Work out the finished part from the listing and answer in its coordinate system (mm). A direction names the side the tool comes from. Give positions to 0.01 mm unless a question says otherwise; leave off trailing zeros. Write each loop counter-clockwise with the first axis right and the second up, starting at its lowest first coordinate (ties: lowest second). Pieces come first, ordered by that corner, then holes. Notation, with made-up numbers: (45.5, 53) - (73.5, 53) arc R4 ccw to (73.5, 59) - close; hole circle Ø5 at (89.25, -13.75). An arc over 180 degrees is marked (long way). Write each question's results on one line, items separated by ' | '. Start each with the question number.
from build123d import *

# Parameters (mm, degrees)
ESQUISSE2_R             = 8.85
ESQUISSE2_R_2           = 8
ENL_V_MAT_EXTRU_1_DEPTH = 8
ESQUISSE3_R             = 1.5
ENL_V_MAT_EXTRU_2_DEPTH = 7
ESQUISSE4_R             = 1
ENL_V_MAT_EXTRU_3_DEPTH = 10
ESQUISSE6_R             = 1
ENL_V_MAT_EXTRU_4_DEPTH = 10
ESQUISSE7_R             = 1
ENL_V_MAT_EXTRU_5_DEPTH = 10


with BuildPart() as part:
    # Esquisse1 → Révolution1 (revolve)
    with BuildSketch(Plane.XY, mode=Mode.PRIVATE) as r_volution1_sk:
        Polygon((2.5, 0), (13.9, 0), (13.9, 1.5), (12.4, 1.5), (12.4, 8), (13.9, 8), (13.9, 9.5), (8.85, 9.5), (8.85, 17.5), (2.5, 17.5), align=None)
    revolve(r_volution1_sk.sketch.rotate(Axis((0, 0, 0), (0, 1, 0)), 90), axis=Axis((0, 0, 0), (0, 1, 0)))

    # Esquisse2 → Enlèv. mat.-Extru.1 (cut)
    with BuildSketch(Plane(origin=(0, 17.5, 0), x_dir=(1, 0, 0), z_dir=(0, 1, 0))):
        Circle(ESQUISSE2_R)
        with Locations(Location((0, 0, 0), (0, 0, 270))):
            Circle(ESQUISSE2_R_2, mode=Mode.SUBTRACT)
    extrude(amount=-ENL_V_MAT_EXTRU_1_DEPTH, mode=Mode.SUBTRACT)

    # Esquisse3 → Enlèv. mat.-Extru.2 (cut)
    with BuildSketch(Plane(origin=(0, 17.5, 0), x_dir=(1, 0, 0), z_dir=(0, 1, 0))):
        with Locations(Location((0, 5.5, 0), (0, 0, 270))):
            Circle(ESQUISSE3_R)
        with Locations(Location((4.763139721, -2.75, 0), (0, 0, 270))):
            Circle(ESQUISSE3_R)
        with Locations(Location((-4.763139721, -2.75, 0), (0, 0, 270))):
            Circle(ESQUISSE3_R)
    extrude(amount=-ENL_V_MAT_EXTRU_2_DEPTH, mode=Mode.SUBTRACT)

    # Esquisse4 → Enlèv. mat.-Extru.3 (cut)
    with BuildSketch(Plane.XY):
        with Locations(Location((0, 13.5, 0), (0, 0, 180))):
            Circle(ESQUISSE4_R)
    extrude(amount=ENL_V_MAT_EXTRU_3_DEPTH, mode=Mode.SUBTRACT)

    # Esquisse6 → Enlèv. mat.-Extru.4 (cut)
    with BuildSketch(Plane(origin=(0, 0, 0), x_dir=(0, 1, 0), z_dir=(0.8660254037844398, 0, 0.499999999999998))):
        with Locations(Location((13.499909745, 0, 0), (0, 0, 270))):
            Circle(ESQUISSE6_R)
    extrude(amount=-ENL_V_MAT_EXTRU_4_DEPTH, mode=Mode.SUBTRACT)

    # Esquisse7 → Enlèv. mat.-Extru.5 (cut)
    with BuildSketch(Plane(origin=(0, 0, 0), x_dir=(0, 1, 0), z_dir=(0.8660254037844364, 0, -0.500000000000004))):
        with Locations(Location((13.5, 0, 0), (0, 0, 90))):
            Circle(ESQUISSE7_R)
    extrude(amount=ENL_V_MAT_EXTRU_5_DEPTH, mode=Mode.SUBTRACT)


solid = part.part
Q1. A cutting plane is placed at C-C, the plane z = -10.75. Write down the section's boundary in (x, y), and give its area (3 significant figures).
Q2. A cutting plane is placed at B-B, the plane y = 8.75. Write down the section's boundary in (x, z), and give its area (3 significant figures).
Q3. Given pin 1 (0.9 mm diameter, centred on x = 5, z = 3, fed in from +Y); pin 2 (2.5 mm diameter, centred on x = 0, y = 13.5, fed in from -Z); pin 3 (4 mm diameter, centred on x = 8, y = 10, fed in from -Z), each flat-ended and moving along its own axis, determine where each tip first touches the part or whether it passes through.
Q4. The mould has two halves that part along X. Classify faces 1 (the cylindrical face through (13.57, 8.76, 3.01)), 2 (the cylindrical face through (3.3, 14.05, 2.42)), 3 (the flat face through (2, 8, -12.4)): pulls with the +X half, pulls with the -X half, needs draft (parallel to the pull), parting line crosses it, or undercut.
Q5. A cutting plane is placed at A-A, the plane x = 0. Write down the section's boundary in (y, z).
Q6. A tool of negligible diameter and unlimited length cuts with its end or side. For faces 4 (the cylindrical face through (0.217, 14.476, 5.106)), 5 (the cylindrical face through (-3.72, 4.8, -11.83)), 6 (the flat face through (0, 10.5, -6)), from which of +Z, -Z, +X, -X, +Y, -Y can it reach the whole face along a straight path? Write none if from no direction.
Q7. Consider L1, parallel to Z at x = -5.25, y = 12.75; L2, parallel to X at y = 13.5, z = 3.75; L3, parallel to X at y = 15, z = 2.75. Determine where each line is inside the solid, lowest interval first.
Q8. A cutting plane is placed at D-D, the plane z = 5. Write down the section's boundary in (x, y) (3 decimals).
Result:
1) outline: (-8.81, 0) - (8.81, 0) - (8.81, 1.5) - (6.18, 1.5) - (6.18, 8) - (8.81, 8) - (8.81, 9.5) - (-8.81, 9.5) - (-8.81, 8) - (-6.18, 8) - (-6.18, 1.5) - (-8.81, 1.5) - close | area: 133 mm2
2) outline: circle Ø27.8 at (0, 0); hole circle Ø5 at (0, 0) | area: 587 mm2
3) pin 1: stops at y = 10.5 | pin 2: stops at z = -8 | pin 3: stops at z = -12.51
4) face 1: parting line crosses it | face 2: undercut | face 3: needs draft
5) outline: (0, -13.9) - (1.5, -13.9) - (1.5, -12.4) - (8, -12.4) - (8, -13.9) - (9.5, -13.9) - (9.5, -8) - (17.5, -8) - (17.5, -7) - (10.5, -7) - (10.5, -4) - (17.5, -4) - (17.5, -2.5) - (0, -2.5) - close; (0, 2.5) - (12.5, 2.5) - (12.5, 8) - (9.5, 8) - (9.5, 13.9) - (8, 13.9) - (8, 12.4) - (1.5, 12.4) - (1.5, 13.9) - (0, 13.9) - close; (14.5, 2.5) - (17.5, 2.5) - (17.5, 8) - (14.5, 8) - close
6) face 4: +Z | face 5: none | face 6: +Y
7) L1: z = -6.04 to -3.79, -2.27 to 1.33, 4.17 to 6.04 | L2: x = -7.07 to -5.88, -3.65 to -1, 1 to 3.65, 5.88 to 7.07 | L3: x = -7.51 to -6.26, -3.26 to 3.26, 6.26 to 7.51
8) outline: (-12.97, 0) - (12.97, 0) - (12.97, 1.5) - (11.347, 1.5) - (11.347, 8) - (12.97, 8) - (12.97, 9.5) - (6.245, 9.5) - (6.245, 17.5) - (-6.245, 17.5) - (-6.245, 9.5) - (-12.97, 9.5) - (-12.97, 8) - (-11.347, 8) - (-11.347, 1.5) - (-12.97, 1.5) - close; hole circle Ø2 at (0, 13.5)
